Could you check a few things on this model? Use its own coordinates, in mm. Face numbers are marked on the shaded views. A direction names the side the tool comes from. Coordinates: 2 decimals unless noted, no trailing zeros. Loops run counter-clockwise (first coordinate to the right, second up) from the corner with the lowest first, then second, coordinate; pieces in that order, holes last. Notation, with made-up numbers: M 66.25,25.5 L 99.25,25.5 A14 cw 99.25,30.5 Z; hole C 35.5,0.25 d4. An arc over 180 degrees is marked long. Write each question's results on one line, items separated by ' | '.
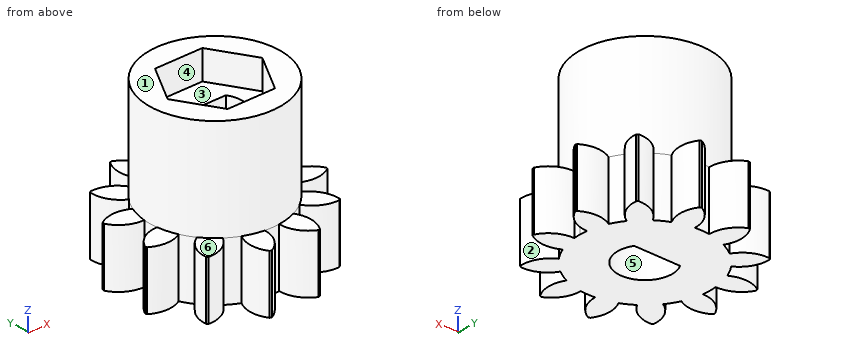
```python
from build123d import *

# Parameters (mm, degrees)
SKETCH1_R           = 6.5
SKETCH1_R_2         = 1
BOSS_EXTRUDE1_DEPTH = 4
CUT_EXTRUDE2_DEPTH  = 5
CIRPATTERN2_COUNT   = 12
SKETCH11_R          = 4.5
BOSS_EXTRUDE2_DEPTH = 11
CUT_EXTRUDE3_START  = 11
CUT_EXTRUDE3_DEPTH  = 2
CUT_EXTRUDE4_DEPTH  = 12


with BuildPart() as part:
    # Sketch1 → Boss-Extrude1 (new body)
    with BuildSketch(Plane.XY):
        Circle(SKETCH1_R)
        Circle(SKETCH1_R_2, mode=Mode.SUBTRACT)
    extrude(amount=BOSS_EXTRUDE1_DEPTH)

    # Sketch4 → Cut-Extrude2 (cut, through all)
    with BuildSketch(Plane.XY):
        with BuildLine():
            ThreePointArc((-0.500194414, 4.472114215), (0, 4.5), (0.500194414, 4.472114215))
            ThreePointArc((0.500194414, 4.472114215), (1.113314535, 5.941215952), (2.604960982, 6.497243899))
            ThreePointArc((2.604960982, 6.497243899), (0, 7), (-2.604960982, 6.497243899))
            ThreePointArc((-2.604960982, 6.497243899), (-1.123395838, 5.950848366), (-0.5, 4.5))
            ThreePointArc((-0.5, 4.5), (-0.500048604, 4.486056768), (-0.500194414, 4.472114215))
        make_face()
    cut_extrude2 = extrude(amount=CUT_EXTRUDE2_DEPTH, mode=Mode.SUBTRACT)

    # CirPattern2: Cut-Extrude2 ×12 about axis
    cirpattern2_axis = Axis((0, 0, 0), (0, 0, 1))
    for i in range(1, CIRPATTERN2_COUNT):
        add(cut_extrude2.rotate(cirpattern2_axis, i * 360 / CIRPATTERN2_COUNT), mode=Mode.SUBTRACT)

    # Sketch11 → Boss-Extrude2 (add)
    with BuildSketch(Plane.XY):
        Circle(SKETCH11_R)
    extrude(amount=BOSS_EXTRUDE2_DEPTH)

    # Sketch12 → Cut-Extrude3 (cut)
    with BuildSketch(Plane.XY.offset(CUT_EXTRUDE3_START)):
        Polygon((3.290896534, 0), (1.645448267, 2.85), (-1.645448267, 2.85), (-3.290896534, 0), (-1.645448267, -2.85), (1.645448267, -2.85), align=None)
    extrude(amount=-CUT_EXTRUDE3_DEPTH, mode=Mode.SUBTRACT)

    # Sketch13 → Cut-Extrude4 (cut, through all)
    with BuildSketch(Plane.XY):
        with BuildLine():
            Line((1.6, 0.95), (-1.6, 0.95))
            ThreePointArc((-1.6, 0.95), (0, -1.860779407), (1.6, 0.95))
        make_face()
    extrude(amount=CUT_EXTRUDE4_DEPTH, mode=Mode.SUBTRACT)


solid = part.part
```
(1) Will these pins go through, and if not, where does the flat tip stop? P1, Ø0.8, axis at x = 1.5, y = 5, coming from the +Z side; P2, Ø3, axis at y = -1.5, z = 6.5, coming from the +X side; P3, Ø5, axis at x = -4, z = 1.5, coming from the -Y side.
Reported:
P1: stops at z = 4 | P2: stops at x = 4.5 | P3: stops at y = -6.3
(2) Imagine slicing it at D-D, the plane y = 1.25. List the corners of the cut face in (x, z) for me.
Reported:
outline: M -6.06,0 L 6.06,0 L 6.06,4 L 4.32,4 L 4.32,11 L 2.57,11 L 2.57,9 L -2.57,9 L -2.57,11 L -4.32,11 L -4.32,4 L -6.06,4 Z
(3) Please list where these lines run through material, in increasing order: probe 1 along Y at (x, z) = (-4, 3.5); probe 2 along Y at (x, z) = (0, 5); probe 3 along Y at (x, z) = (0.5, 10.75). Write a range as from..to.
Reported:
probe 1: y = -4.6..-2.94, -2.06..2.06, 2.94..4.6 | probe 2: y = -4.5..-1.86, 0.95..4.5 | probe 3: y = -4.47..-2.85, 2.85..4.47
(4) Which directions (+Z, -Z, +X, -X, +Y, -Y) give clear straight access to the entire face, cutting with the end or side of a thin tool? Please do the marked faces 4, 5 and 6.
Reported:
face 4: +Z | face 5: +Z, -Z | face 6: +Z, -X, -Y
(5) Imagine slicing it at A-A, the plane x = 1.25. List the corners of the cut face in (y, z) for me.
Reported:
outline: M -6.06,0 L -1.38,0 L -1.38,9 L -2.85,9 L -2.85,11 L -4.32,11 L -4.32,4 L -6.06,4 Z; M 0.95,0 L 6.06,0 L 6.06,4 L 4.32,4 L 4.32,11 L 2.85,11 L 2.85,9 L 0.95,9 Z
(6) Imagine slicing it at C-C, the plane y = -5.25. List the corners of the cut face in (x, z) for me.
Reported:
outline: M -2.08,0 L -0.65,0 L -0.65,4 L -2.08,4 Z; M 0.65,0 L 2.08,0 L 2.08,4 L 0.65,4 Z
(7) Imagine slicing it at B-B, the plane z = 10.25. List the corners of the cut face in (x, y) for me, and give its area (3 significant figures).
Reported:
outline: C 0,0 d9; hole M -3.29,0 L -1.65,-2.85 L 1.65,-2.85 L 3.29,0 L 1.65,2.85 L -1.65,2.85 Z | area: 35.5 mm2
(8) If we mould it in two halves opening along X, with no side actions, what happens to the marked faces 1, 2 and 3? For each: released by +X, released by -X, zero draft, split by the parting line, or undercut.
Reported:
face 1: zero draft | face 2: released by +X | face 3: undercut
